Input: part model. Units: mm. Frame: model coordinates. Face numbers are marked on the shaded views. A direction names the side the tool comes from. Round coordinates to 2 decimals unless told otherwise and drop trailing zeros. Order: outer loops, then holes, each group sorted by start corner. A loop starts at its lowest first (then second) coordinate and runs counter-clockwise, first axis right, second up. Notation, with made-up numbers: (20, 64) - (49, 64) arc R30 cw to (49, 93) - close; hole circle Ø1 at (-36, -14). An arc over 180 degrees is marked (long way). One line per item, written item: value. Start each with the question number.
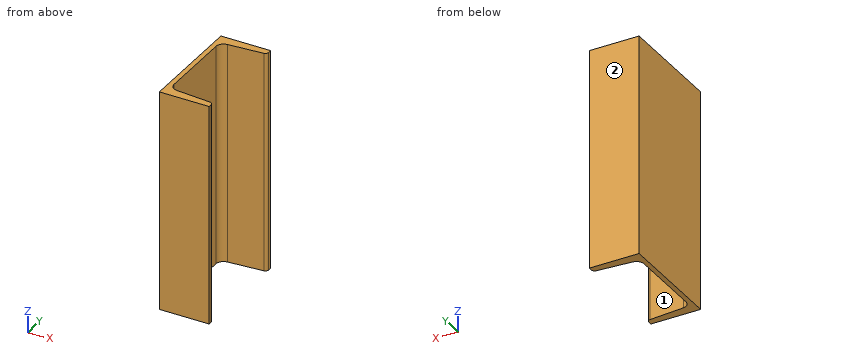
Autodesk Inventor part; units mm, degrees
ref_plane "Начальная плоскость" through (0, 0, 23) normal (0, 0, 1) x (1, 0, 0)
ref_plane "Конечная плоскость" through (0, 0, 227) normal (0, 0, 1) x (1, 0, 0)
ref_plane "РабПлоскость8" through (-82, -50, 23) normal (0, 0, -1) x (-1, 0, 0)
ref_plane "Начальная плоскость" through (0, 0, 23) normal (0, 0, 1) x (1, 0, 0)
ref_plane "Конечная плоскость" through (0, 0, 227) normal (0, 0, 1) x (1, 0, 0)
sketch "Эскиз" plane through (0, 0, 0) normal (0, 0, 1) x (1, 0, 0)
  line L0 (46, -50) -> (0, -50)
  line L1 (46, -50) -> (46, -46.6496)
  line L2 (43.2392, -43.6591) -> (10.9418, -41.0753)
  line L3 (4.5, -34.0976) -> (4.5, 34.0976)
  line L4 (43.2392, 43.6591) -> (10.9418, 41.0753)
  line L5 (46, 46.6496) -> (46, 50)
  line L6 (0, 50) -> (46, 50)
  line L7 (0, -50) -> (0, 50)
  arc A0 (4.5, -34.0976) -> (10.9418, -41.0753) centre (11.5, -34.0976) ccw
  arc A1 (10.9418, 41.0753) -> (4.5, 34.0976) centre (11.5, 34.0976) ccw
  arc A2 (46, -46.6496) -> (43.2392, -43.6591) centre (43, -46.6496) ccw
  arc A3 (43.2392, 43.6591) -> (46, 46.6496) centre (43, 46.6496) ccw
  line L8 (0, 70) -> (0, -70) construction
  line L9 (-9.3169, 0) -> (55.9016, 0) construction
  point P0 (46, -43.88)
  point P1 (4.5, -40.56)
  point P2 (4.5, 40.56)
  point P3 (46, 43.88)
  dimension "d3" = 46
  dimension "d5" = 4.5
  dimension "d7" = 100
  dimension "d9" = 9.44
  dimension "d11" = 9.44
  dimension "d13" = 6.12
  dimension "d15" = 6.12
  dimension "d22" = 7
  dimension "d23" = 3
  dimension "d24" = 50
  dimension "d25" = 0
extrude "Тело" add sketch "Эскиз" along normal up to surface (204 mm away) from surface at 23
sketch "Sketch3" plane through (0, 0, 0) normal (0, 0, 1) x (1, 0, 0)
  line L0 (0, 0) -> (10, 0)
ref_plane "Work Plane7" through (0, 0, 0) normal (0, -1, 0) x (1, 0, 0)
sketch "Sketch4" plane through (0, 0, 0) normal (0, -1, 0) x (1, 0, 0)
  line L0 (-2, 23) -> (12, 23)
  line L1 (-2, 227) -> (12, 227)
  dimension "d29" = 204
ref_plane "РабПлоскость8" through (-82, -50, 23) normal (0, 0, -1) x (-1, 0, 0)
split "Разделение1" plane through (-82, -50, 23) removes the side toward (0, 0, -1)
ref_plane "РабПлоскость9" through (368, -50, 227) normal (0, 0, 1) x (1, 0, 0)
split "Разделение2" plane through (368, -50, 227) removes the side toward (0, 0, 1)
equation "\"d3\" = b"
equation "\"d7\" = ParH"
equation "\"d22\" = R"
equation "\"d23\" = R1"
equation "\"d24\" = 0.5 * d7"
equation "\"d16\" = G_L"
equation "\"R1\" = 3"
equation "\"R\" = 7"
equation "\"t1\" = 4.5"
equation "\"t2\" = 7.6"
equation "\"ParH\" = 100"
equation "\"b\" = 46"
equation "\"msp_x1\" = 0.04 * b"
equation "\"msp_x2\" = -0.08 * t1 + 0.04 * b"
equation "\"G_L\" = d29"
equation "\"ex\" = 0"
equation "\"G_OFFSET_START\" = -23"
equation "\"G_OFFSET_END\" = -23"
equation "\"d26\" = -G_OFFSET_START"
equation "\"d27\" = G_OFFSET_END + B_L"
properties part number "Швеллер 10U-204 ГОСТ 8240-97" material "Сталь, мягкая, сварочная"
1. Pin query (flat end, axial travel): pin 1 (8 mm diameter, centred on y = -2, z = 148.5, fed in from +X). Return the tip coordinate at first contact, or that it passes through.
2. Section D-D (y = 27.5). Return the cut outline in (x, z), then the cut area to 3 significant figures.
3. Section B-B (z = 161). Return the cut outline in (x, y).
4. Set-up query: the marked faces 1 and 2. Return all of +Z, -Z, +X, -X, +Y, -Y with unobstructed straight access to the full face (end or side cutting, diameter ignored); none if empty.
5. Line query: line 1 (Y direction, x = 21, z = 166.5); line 2 (Y direction, x = 35.5, z = 217); line 3 (X direction, y = -4.5, z = 175.5). Output: solid intervals per line, ascending. Write a range as from..to.
6. Section A-A (x = 37). Return the cut outline in (y, z).
7. Section C-C (x = 17.5). Return the cut outline in (y, z).
Solved:
1. pin 1: stops at x = 4.5
2. outline: (0, 23) - (4.5, 23) - (4.5, 227) - (0, 227) - close
2. area: 918 mm²
3. outline: (0, -50) - (46, -50) - (46, -46.65) arc R3 ccw to (43.24, -43.66) - (10.94, -41.08) arc R7 cw to (4.5, -34.1) - (4.5, 34.1) arc R7 cw to (10.94, 41.08) - (43.24, 43.66) arc R3 ccw to (46, 46.65) - (46, 50) - (0, 50) - close
4. face 1: +Z, -Z, +X
4. face 2: +Z, -Z, +X, -X, +Y
5. line 1: y = -50..-41.88, 41.88..50
5. line 2: y = -50..-43.04, 43.04..50
5. line 3: x = 0..4.5
6. outline: (-50, 23) - (-43.16, 23) - (-43.16, 227) - (-50, 227) - close; (43.16, 23) - (50, 23) - (50, 227) - (43.16, 227) - close
7. outline: (-50, 23) - (-41.6, 23) - (-41.6, 227) - (-50, 227) - close; (41.6, 23) - (50, 23) - (50, 227) - (41.6, 227) - close
